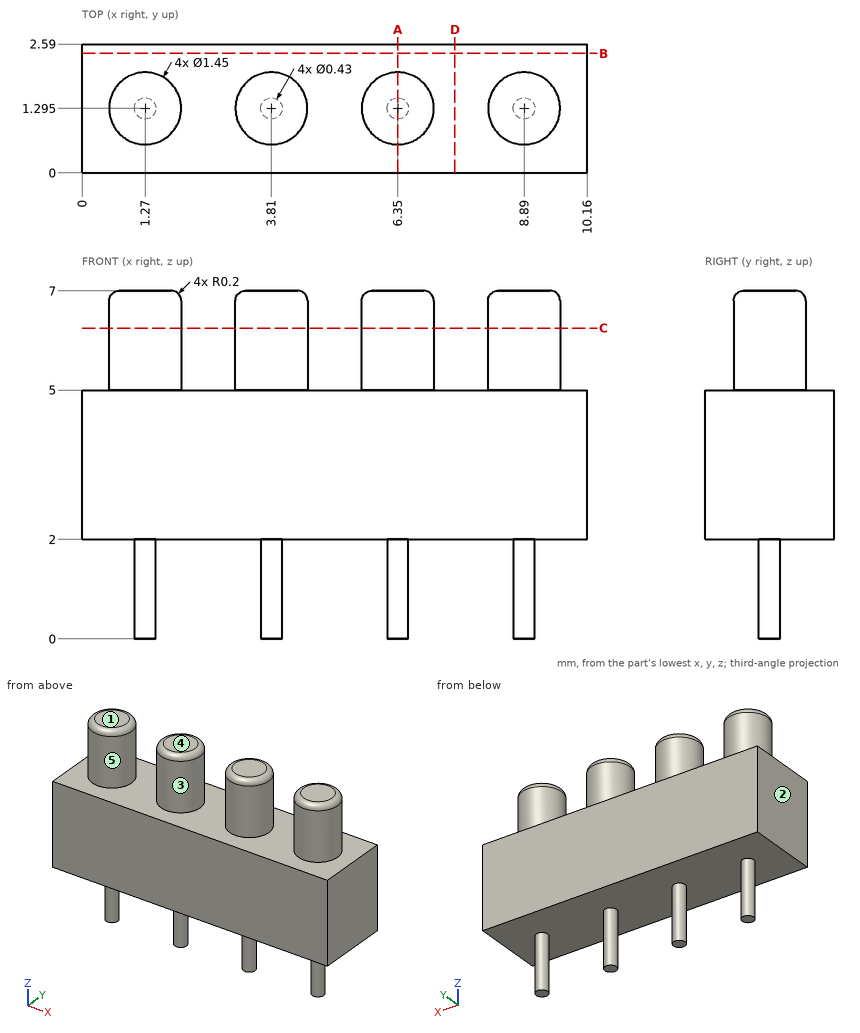
The drawing under review shows one solid part. Ordinate dimensions are in mm from its lowest x, y, z. A direction names the side the tool comes from. Round coordinates to 2 decimals unless told otherwise and drop trailing zeros. Write each loop counter-clockwise with the first axis right and the second up, starting at its lowest first coordinate (ties: lowest second). Pieces come first, ordered by that corner, then holes. Notation, with made-up numbers: M 50,-34.75 L 63,-34.75 A17 ccw 63,-6.75 Z; hole C 21,47 d4. An arc over 180 degrees is marked long. One line per item, written item: value. Start each with the question number.
(1) We need section A-A (x = 6.35). Give the boundary of the cut face in (y, z), and give its area (3 significant figures).
(2) We need section B-B (y = 2.4). Give the boundary of the cut face in (x, z), and give its area (3 significant figures).
(3) Wall thickness on line 1 (X direction, y = 0.85, z = 5.75); line 2 (Z direction, x = 9.5, y = 2.1); line 3 (Z direction, x = 1.25, y = 0.8): over which ranges is each line inside the solid? List them lowest first.
(4) We need section C-C (z = 6.25). Give the boundary of the cut face in (x, y) (3 decimals).
(5) We need section D-D (x = 7.5). Give the boundary of the cut face in (y, z).
(6) Insertion check: pin 1 (1 mm diameter, centred on x = 3, y = 2, fed in from +Z); pin 2 (1.3 mm diameter, centred on x = 5, y = 1, fed in from -Z). Each pin has a flat end and moves straight along its axis. Give the tip position at first contact, or say it passes through.
(7) The part is to be moulded in two halves that separate along X. For the marked faces 1, 2 and 3, say which applies: released by +X, released by -X, zero draft, split by the parting line, or undercut.
(8) Machinability: for the marked faces 4 and 5, which of the approach directions +Z, -Z, +X, -X, +Y, -Y give a long, thin tool a straight path to every point of the face, cutting with its end or side? Answer none if there is none.
Result:
1. outline: M 0,2 L 1.08,2 L 1.08,0 L 1.51,0 L 1.51,2 L 2.59,2 L 2.59,5 L 2.02,5 L 2.02,6.8 A0.2 ccw 1.82,7 L 0.77,7 A0.2 ccw 0.57,6.8 L 0.57,5 L 0,5 Z
1. area: 11.5 mm²
2. outline: M 0,2 L 10.16,2 L 10.16,5 L 0,5 Z
2. area: 30.5 mm²
3. line 1: 0.7 to 1.84, 3.24 to 4.38, 5.78 to 6.92, 8.32 to 9.46
3. line 2: 2 to 5
3. line 3: 2 to 7
4. outline: C 1.27,1.295 d1.45; C 3.81,1.295 d1.45; C 6.35,1.295 d1.45; C 8.89,1.295 d1.45
5. outline: M 0,2 L 2.59,2 L 2.59,5 L 0,5 Z
6. pin 1: z = 6.99
6. pin 2: z = 2
7. face 1: zero draft
7. face 2: released by -X
7. face 3: undercut
8. face 4: +Z, +X, -X, +Y, -Y
8. face 5: +Z
